Build history of the part. All positions in model axes, mm. Face numbers are marked on the shaded views. Give positions to 0.01 mm unless a question says otherwise; leave off trailing zeros. Order: outer loops, then holes, each group sorted by start corner. A loop starts at its lowest first (then second) coordinate and runs counter-clockwise, first axis right, second up. Notation, with made-up numbers: M 56.25,-13.75 L 100.25,-13.75 A21 cw 100.25,25.25 Z; hole C 22,-28 d6. An arc over 180 degrees is marked long. One line per item, written item: value.
Autodesk Fusion 360 part; units mm, degrees
sketch "Sketch1" plane through (0, 0, 0) normal (1, 0, 0) x (0, 1, 0)
  line L0 (0, 0) -> (12, 0)
  line L1 (12, 0) -> (12, 10)
  line L2 (12, 10) -> (0, 10)
  line L3 (0, 10) -> (0, 0)
  circle A0 centre (8, 5) radius 2
  dimension "d3" = 12
  dimension "d4" = 4
extrude "Extrude1" add sketch "Sketch1" along normal blind 4 contours L0 L1 L2 L3 | A0 makes body 1
extrude "Extrude2" add sketch "Sketch1" along normal blind 4 separate body makes body 2
extrude "Extrude4" cut sketch "Sketch1" along normal blind 125 contours A0 bodies 1
sketch "Sketch3" plane through (0, 6, 5) normal (1, 0, 0) x (0, 1, 0)
  line L0 (-6, 5) -> (-2, 5)
  line L1 (-2, 5) -> (-2, -5)
  line L2 (-6, -5) -> (-6, 5)
  line L3 (-2, -5) -> (-6, -5)
extrude "Extrude5" add sketch "Sketch3" along normal blind 80 bodies 1 2
sketch "Sketch4" plane through (0, 4, 0) normal (0, 1, 0) x (-1, 0, 0)
  line L0 (-4, 0) -> (-4, 10)
  line L1 (-4, 10) -> (-80, 10)
  line L2 (-80, 10) -> (-80, 0)
  line L3 (-80, 0) -> (-4, 0)
  circle A0 centre (-42, 5) radius 2
extrude "Extrude6" cut sketch "Sketch4" against normal blind 14 contours A0 bodies 1
sketch "Sketch5" plane through (0, 0, 10) normal (0, 0, 1) x (-1, 0, 0)
  line L0 (-4, -4) -> (-4, -12)
  line L1 (-4, -12) -> (0, -12)
  line L2 (0, -12) -> (0, 0)
  line L3 (0, 0) -> (-80, 0)
  line L4 (-80, 0) -> (-80, -4)
  line L5 (-80, -4) -> (-4, -4)
  line L6 (-80, 0) -> (-84, 0)
  line L7 (-84, 0) -> (-84, -12)
  line L8 (-84, -12) -> (-80, -12)
  line L9 (-80, -12) -> (-80, 0)
  dimension "d15" = 4
extrude "Extrude7" add sketch "Sketch5" against normal blind 10 contours L4 L6 L7 L8 L9 bodies 1
extrude "Extrude8" cut sketch "Sketch1" along normal blind 360 contours A0 bodies 1
sketch "Sketch6" plane through (0, 4, 0) normal (0, 1, 0) x (-1, 0, 0)
  circle A0 centre (-42, 5) radius 2
  line L0 (-4, 0) -> (-4, 10)
  line L1 (-4, 10) -> (-80, 10)
  line L2 (-80, 10) -> (-80, 0)
  line L3 (-80, 0) -> (-4, 0)
  circle A1 centre (-42, 5) radius 5
  line L4 (-42, 5) -> (-40, 5)
  line L5 (-37, 5) -> (-47, 5)
  line L6 (-37, 5) -> (-37.5116, 6.9335)
  line L7 (-47, 5) -> (-46.4882, 6.9334)
  line L8 (-47, 5) -> (-46.6078, 3.0388)
  line L9 (-37, 5) -> (-37.5177, 3.0682)
  line L10 (-46.4882, 6.9334) -> (-80, 10)
  line L11 (-46.6078, 3.0388) -> (-80, 0)
  line L12 (-37.5116, 6.9335) -> (-4, 10)
  line L13 (-37.5177, 3.0682) -> (-4, 0)
  dimension "d20" = 2
  dimension "d21" = 2
  dimension "d22" = 2
  dimension "d23" = 2
extrude "Extrude9" cut sketch "Sketch6" against normal blind 20 contours L1 A1 L12 | L3 A1 L13 | L1 A1 L10 | L3 A1 L8 L11 bodies 1
fillet "Fillet1" radius 2.5 4 edges at (0, 0, 5) (84, 0, 5) (80, 4, 5) (4, 4, 5) on bodies 1
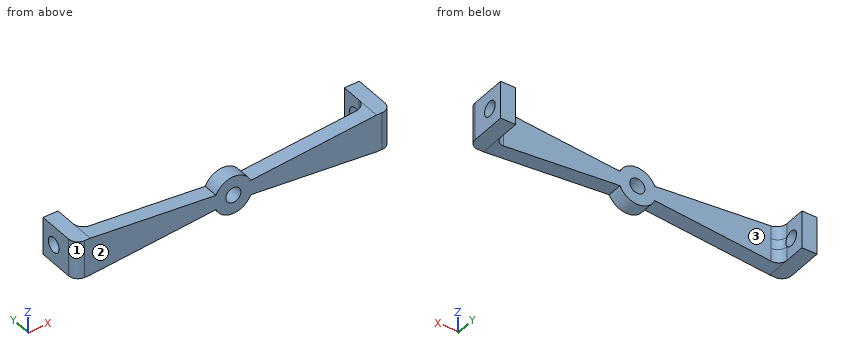
1) Drill centre lines: probe 1 along X at (y, z) = (10, 8.5); probe 2 along Z at (x, y) = (82.15, 8); probe 3 along Y at (x, z) = (80.9, 5). Where is each one in solid material? Low to high. Write a range as from..to.
Check values:
probe 1: 0..4, 80..84
probe 2: 0..3, 7..10
probe 3: 0..6, 10..12
2) Pin check, flat tips, straight feed: pin 1 (3 mm diameter, centred on x = 42, z = 5, fed in from -Y); pin 2 (2 mm diameter, centred on x = 38, y = 1.5, fed in from -Z); pin 3 (5 mm diameter, centred on x = 29.5, z = 3, fed in from +Y). Stop position of each tip, or through.
Check values:
pin 1: through
pin 2: z = 1
pin 3: y = 4
3) Saw through at A-A, the plane y = 11. Write the cut outline in (x, z), then the cut area to 3 significant figures.
Check values:
outline: M 0,0 L 4,0 L 4,10 L 0,10 Z; M 80,0 L 84,0 L 84,10 L 80,10 Z
area: 80.0 mm^2
4) Saw through at B-B, the plane x = 42. Write the cut outline in (y, z).
Check values:
outline: M 0,0 L 4,0 L 4,3 L 0,3 Z; M 0,7 L 4,7 L 4,10 L 0,10 Z
5) Mould opens along X. For the marked faces 1, 2 and 3 say: released by +X, released by -X, zero draft, split by the parting line, or undercut.
Check values:
face 1: released by -X
face 2: zero draft
face 3: undercut
6) Saw through at D-D, the plane z = 5. Give the number of separate pieces and of enclosed holes in the cut face, then the cut area to 3 significant figures.
Check values:
separate pieces: 4
enclosed holes: 0
area: 352 mm^2
7) Saw through at C-C, the plane y = 8. Write the cut outline in (x, z), then the cut area to 3 significant figures.
Check values:
outline: M 0,0 L 4,0 L 4,3 L 0,3 Z; M 0,7 L 4,7 L 4,10 L 0,10 Z; M 80,0 L 84,0 L 84,3 L 80,3 Z; M 80,7 L 84,7 L 84,10 L 80,10 Z
area: 48.0 mm^2
